The model under review builds one solid part; all positions refer to its coordinate system, in mm. A direction names the side the tool comes from. Coordinates: 2 decimals unless noted, no trailing zeros. Order: outer loops, then holes, each group sorted by start corner. A loop starts at its lowest first (then second) coordinate and runs counter-clockwise, first axis right, second up. Notation, with made-up numbers: (49, 17.5) - (108, 17.5) arc R21 cw to (108, 27.5) - close; hole circle Ø9 at (15.5, 9). An arc over 180 degrees is marked (long way). Answer in a Markdown table with one row per item.
```python
from build123d import *

# Parameters (mm, degrees)
FILLET2_R                = 3
BOSS_EXTRUDE1_DEPTH      = 25
BOSS_EXTRUDE1_DEPTH_BACK = 25
SKETCH3_R                = 4.875
SKETCH2_R                = 4.5
CUT_EXTRUDE2_DEPTH       = 120
FILLET3_R                = 1


with BuildPart() as part:
    # Sketch1 → Revolve1 (revolve)
    with BuildSketch(Plane(origin=(0, 0, 0), x_dir=(0, 0, -1), z_dir=(1, 0, 0)), mode=Mode.PRIVATE) as revolve1_sk:
        with BuildLine():
            Line((0, 12.5), (-40, 12.5))
            Line((-40, 12.5), (-40, 10))
            Line((-40, 10), (-62, 10))
            Line((-62, 10), (-62, 7.5))
            Line((-62, 7.5), (-132, 7.5))
            Line((-132, 7.5), (-132, 0))
            Line((-132, 0), (12.5, 0))
            ThreePointArc((12.5, 0), (8.838834765, 8.838834765), (0, 12.5))
        make_face()
    revolve(revolve1_sk.sketch.rotate(Axis((0, 0, 132), (0, 0, -1)), 90), axis=Axis((0, 0, 132), (0, 0, -1)))

    # Fillet2
    # the kernel refuses this fillet: 3 mm, written as the material it takes off along each edge
    with BuildSketch(Plane(origin=(0, 0, 40), x_dir=(1, 0, 0), z_dir=(0, 1, 0))) as fillet2_piece_1:
        with BuildLine():
            CenterArc((9.5, 2.958039892), FILLET2_R, 279.594068227, 80.405931773)
            Line((10, 0), (10.01, -0.059160798))
            ThreePointArc((10.01, -0.059160798), (11.25, -0.06), (12.5, -0.06))
            Line((12.5, -0.06), (12.56, 0))
            Line((12.56, 0), (12.56, 2.958039892))
            Line((12.56, 2.958039892), (12.5, 2.958039892))
        make_face()
    revolve(axis=Axis((0, 0, 40), (0, 0, -1)), mode=Mode.SUBTRACT)
    with BuildSketch(Plane(origin=(0, 0, 62), x_dir=(1, 0, 0), z_dir=(0, 1, 0))) as fillet2_piece_2:
        with BuildLine():
            CenterArc((7, 2.958039892), FILLET2_R, 279.594068227, 80.405931773)
            Line((7.5, 0), (7.51, -0.059160798))
            ThreePointArc((7.51, -0.059160798), (8.75, -0.06), (10, -0.06))
            Line((10, -0.06), (10.06, 0))
            Line((10.06, 0), (10.06, 2.958039892))
            Line((10.06, 2.958039892), (10, 2.958039892))
        make_face()
    revolve(axis=Axis((0, 0, 62), (0, 0, -1)), mode=Mode.SUBTRACT)

    # Sketch3 → Boss-Extrude1 (add, two sides: drawn at the far end of the back side and taken through both)
    with BuildSketch(Plane(origin=(0, 0, 0), x_dir=(0, 0, -1), z_dir=(1, 0, 0)).offset(-BOSS_EXTRUDE1_DEPTH_BACK)):
        with Locations((-30.171572875, -0.635390854)):
            Circle(SKETCH3_R)
    extrude(amount=BOSS_EXTRUDE1_DEPTH + BOSS_EXTRUDE1_DEPTH_BACK)

    # Sketch2 → Cut-Extrude2 (cut)
    with BuildSketch(Plane.XY.offset(132)):
        Circle(SKETCH2_R)
    extrude(amount=-CUT_EXTRUDE2_DEPTH, mode=Mode.SUBTRACT)

    # Fillet3
    fillet3_edges = [part.edges().sort_by_distance(p)[0] for p in [
        (-7.5, 0, 132),
    ]]
    fillet(fillet3_edges, radius=FILLET3_R)


solid = part.part
```
Item 1: We need section A-A, the plane x = 0. Write out the cut boundary in (y, z), then the cut area to 3 significant figures.
Check values:
| item | result |
|---|---|
| outline | (-12.5, 0) arc R12.5 ccw to (12.5, 0) - (12.5, 37.04) arc R3 ccw to (10, 40) - (10, 59.04) arc R3 ccw to (7.5, 62) - (7.5, 131) arc R1 ccw to (6.5, 132) - (4.5, 132) - (4.5, 12) - (-4.5, 12) - (-4.5, 132) - (-6.5, 132) arc R1 ccw to (-7.5, 131) - (-7.5, 62) arc R3 ccw to (-10, 59.04) - (-10, 40) arc R3 ccw to (-12.5, 37.04) - close |
| area | 1,650 mm^2 |
Item 2: We need section D-D, the plane x = -20.5. Write out the cut boundary in (y, z) (3 decimals), then the cut area to 3 significant figures.
Check values:
| item | result |
|---|---|
| outline | circle Ø9.75 at (-0.635, 30.172) |
| area | 74.7 mm^2 |
Item 3: Tool access review of faces 4 (the face through (-18.2, -5.4, 31.2)), 5 (the face through (25, -1, 30)), 6 (the face through (-25, -1, 30)), 7 (the face through (-10, 0, 50)), 8 (the face through (18, -5.4, 31.2)): name each direction out of +Z, -Z, +X, -X, +Y, -Y from which nothing blocks a thin tool from reaching the whole face with its end or side.
Check values:
| item | result |
|---|---|
| face 4 | -X |
| face 5 | +Z, -Z, +X, +Y, -Y |
| face 6 | +Z, -Z, -X, +Y, -Y |
| face 7 | +Z |
| face 8 | +X |
Item 4: We need section B-B, the plane z = 27.5. Write out the cut boundary in (x, y), then the cut area to 3 significant figures.
Check values:
| item | result |
|---|---|
| outline | (-25, -4.71) - (-11.58, -4.71) arc R12.5 ccw to (11.58, -4.71) - (25, -4.71) - (25, 3.44) - (12.02, 3.44) arc R12.5 ccw to (-12.02, 3.44) - (-25, 3.44) - close; hole circle Ø9 at (0, 0) |
| area | 635 mm^2 |
Item 5: We need section C-C, the plane z = 105.5. Write out the cut boundary in (x, y).
Check values:
| item | result |
|---|---|
| outline | circle Ø15 at (0, 0); hole circle Ø9 at (0, 0) |
Item 6: Mouldability with a two-part tool opening along Y and no side actions: class faces 1 (the face through (0, 0, 12)), 2 (the face through (4.032, -6.324, 96.983)), 3 (the face through (-1.54, -4.42, 132)) as +Y half, -Y half, draft (parallel to the pull), parting line (faces both ways), or undercut.
Check values:
| item | result |
|---|---|
| face 1 | undercut |
| face 2 | parting line |
| face 3 | draft |
Item 7: Clearance check with flat-ended pins moving along their axes: pin 1 Ø8 at (x, y) = (0, 0) entering from +Z; pin 2 Ø1 at (y, z) = (-7, 60.5) entering from +X; pin 3 Ø8 at (x, y) = (19, -4) entering from +Z. State where each tip first meets the part, or that it passes through.
Check values:
| item | result |
|---|---|
| pin 1 | z = 12 |
| pin 2 | x = 7.2 |
| pin 3 | z = 35.05 |
Item 8: To check wall thickness, follow line 1 (Y direction, x = 0, z = 91); line 2 (X direction, y = 0.5, z = 25); line 3 (Y direction, x = 0, z = 41.5). State the ranges of each line that lie inside material, in increasing order. Write a range as from..to.
Check values:
| item | result |
|---|---|
| line 1 | -7.5..-4.5, 4.5..7.5 |
| line 2 | -12.49..-4.47, 4.47..12.49 |
| line 3 | -10..-4.5, 4.5..10 |
